Autodesk Inventor part; units mm, degrees
ref_plane "YZ Plane" through (0, 0, 0) normal (1, 0, 0) x (0, 1, 0)
ref_plane "XZ Plane" through (0, 0, 0) normal (0, 1, 0) x (-1, 0, 0)
ref_plane "XY Plane" through (0, 0, 0) normal (0, 0, 1) x (1, 0, 0)
sketch "Sketch1" plane through (0, 0, 0) normal (0, 1, 0) x (-1, 0, 0)
  line L0 (0, 0) -> (7, 0)
  line L1 (7, 0) -> (7, -150)
  line L2 (7, -150) -> (0, -150)
  line L3 (0, -150) -> (0, -146)
  line L4 (0, -146) -> (3, -146)
  line L5 (3, -146) -> (3, -4)
  line L6 (3, -4) -> (0, -4)
  line L7 (0, -4) -> (0, 0)
  dimension "d4" = 7
  dimension "d5" = 3
  dimension "d6" = 4
  dimension "d7" = 150
sketch "Sketch2" plane through (0, 0, 0) normal (0, 0, 1) x (1, 0, 0)
  line L0 (0, 0) -> (0, 95.438)
  line L1 (0, 95.438) -> (49.962, 145.4)
  dimension "d8" = 135
  dimension "d9" = 95.438
  dimension "d10" = 70.657
sweep "Sweep1" add profiles "Sketch1" path "Sketch2"
sketch "Sketch3" plane through (45.0123, 150.3498, -150) normal (0.7071, 0.7071, 0) x (-0.7071, 0.7071, 0)
  line L0 (-7, 150) -> (-7, 146)
  line L1 (-74.4849, 4) -> (-7, 4)
  line L2 (-7, 146) -> (-7, 4)
  line L3 (-72.3635, 146) -> (-4, 146)
  line L4 (-7, 146) -> (-4, 146)
  line L5 (-4, 4) -> (-7, 4)
  line L6 (-4, 146) -> (-4, 4)
  line L7 (-4, 4) -> (-7, 4)
  point P0 (-74.4849, 150)
extrude "Extrusion1" add sketch "Sketch3" against normal blind 5.657
sketch "Sketch5" plane through (-7, 0, 0) normal (0, -1, 0) x (1, 0, 0)
  line L0 (4, -4) -> (4, -146)
  line L1 (7, -4) -> (4, -4)
  line L2 (4, -146) -> (7, -146)
  line L3 (7, -146) -> (7, -4)
  line L4 (7, -146) -> (7, -150)
  point P0 (7, 0)
extrude "Extrusion2" add sketch "Sketch5" against normal blind 4
sketch "Sketch6" plane through (-7, 98.3375, -150) normal (-0.7071, 0.7071, 0) x (-0.7071, -0.7071, 0)
  line L0 (-16.7782, 123.5) -> (-56.7782, 123.5)
  line L1 (-56.7782, 123.5) -> (-56.7782, 26.5)
  line L2 (-56.7782, 26.5) -> (-16.7782, 26.5)
  line L3 (-16.7782, 26.5) -> (-16.7782, 123.5)
  line L4 (0, 0) -> (0, 150)
  line L5 (0, 0) -> (-73.5565, 0)
  point P0 (64.5854, 150)
  point P1 (-16.7782, 75)
  point P2 (0, 75)
  point P3 (-36.7782, 26.5)
  point P4 (-36.7782, 0)
  dimension "d17" = 97
  dimension "d18" = 40
extrude "Extrusion3" cut sketch "Sketch6" against normal blind 4
properties part number "lid"
The listing builds one solid part. Answer for the finished solid, in the listing's coordinates (mm). A direction names the side the tool comes from. Coordinates: 2 decimals unless noted, no trailing zeros. Order: outer loops, then holes, each group sorted by start corner. A loop starts at its lowest first (then second) coordinate and runs counter-clockwise, first axis right, second up.
Q1. Which of the six approach directions +Z, -Z, +X, -X, +Y, -Y give full straight-line access (tool end or side, diameter ignored) to faces 5 (the face through (-2, 81, -150)), 6 (the face through (0, 2, -75)), 7 (the face through (-3, 51, -74))?
Q2. A cutting plane is placed at B-B, the plane y = 122. Write down the section's boundary in (x, z), and give its area (3 significant figures).
Q3. Given P1, Ø2.5, axis at x = -1.5, z = -108.5, coming from the +Y side; P2, Ø6, axis at x = 38.5, z = -79.5, coming from the +Y side; P3, Ø6, axis at y = 90.5, z = -72.5, coming from the +X side; P4, Ø14.5, axis at x = 12, y = 41, coming from the +Z side, each flat-ended and moving along its own axis, determine where each tip first touches the part or whether it passes through.
Q4. For a pull along Y with two mould halves and no side action, classify faces 1 (the face through (-0.2, 74.1, -4)), 2 (the face through (20, 123, -26.5)), 3 (the face through (2.03, 107.37, -76.05)), 4 (the face through (47.3, 142.74, -69.09)) as pulls with the +Y half, pulls with the -Y half, needs draft (parallel to the pull), parting line crosses it, or undercut.
Q5. A cutting plane is placed at D-D, the plane x = 16. Write down the section's boundary in (y, z), and give its area (3 significant figures).
Q6. A cutting plane is placed at C-C, the plane y = 50. Write down the section's boundary in (x, z).
Q7. Consider line 1 (X direction, y = 43, z = -125); line 2 (Y direction, x = 19.5, z = -139); line 3 (Y direction, x = 37.5, z = -67). Determine where each line is inside the solid, lowest interval first.
Answers follow:
1. face 5: -Z, +X, -X, +Y, -Y
1. face 6: +Z, -Z, +X, -Y
1. face 7: +X
2. outline: (16.66, -150) - (26.56, -150) - (26.56, -146) - (22.32, -146) - (22.32, -123.5) - (16.66, -123.5) - close; (16.66, -26.5) - (22.32, -26.5) - (22.32, -4) - (26.56, -4) - (26.56, 0) - (16.66, 0) - close
2. area: 334 mm2
3. P1: stops at y = 105.09
3. P2: stops at y = 146.84
3. P3: stops at x = -3
3. P4: passes through
4. face 1: undercut
4. face 2: needs draft
4. face 3: pulls with the +Y half
4. face 4: pulls with the -Y half
5. outline: (111.44, -150) - (121.34, -150) - (121.34, -123.5) - (115.68, -123.5) - (115.68, -146) - (111.44, -146) - close; (111.44, -4) - (115.68, -4) - (115.68, -26.5) - (121.34, -26.5) - (121.34, 0) - (111.44, 0) - close
5. area: 334 mm2
6. outline: (-7, -150) - (0, -150) - (0, -146) - (-3, -146) - (-3, -4) - (0, -4) - (0, 0) - (-7, 0) - close
7. line 1: x = -7 to -3
7. line 2: y = 119.18 to 124.84
7. line 3: y = 137.18 to 142.84
